from build123d import *

# Parameters (mm, degrees)
F1_DEPTH       = 10
F2_R           = 4.5
F3_R           = 1
F4_DEPTH       = 4
F5_R           = 2.4
F6_DEPTH       = 7.5
F3_R_2         = 2.4
F7_DEPTH       = 25
F7_DEPTH_BACK  = 25
F8_R           = 5
F9_R           = 1
F9_R_2         = 1.9
F10_DEPTH      = 25
F10_DEPTH_BACK = 25
F11_R          = 1


with BuildPart() as f1:
    # F0 (on Top) → F1 (new body)
    with BuildSketch(Plane.XY):
        Polygon((-22.5, 0), (0, 0), (22.5, 0), (22.5, 28.5), (19, 28.5), (19, 3.5), (0, 3.5), (-19, 3.5), (-19, 28.5), (-22.5, 28.5), align=None)
    extrude(amount=F1_DEPTH)

    # F2
    f2_edges = [f1.edges().sort_by_distance(p)[0] for p in [
        (-20.75, 28.5, 10),
        (-20.75, 28.5, 0),
        (20.75, 28.5, 10),
        (20.75, 28.5, 0),
    ]]
    fillet(f2_edges, radius=F2_R)

    # F3 (on face) → F4 (cut)
    with BuildSketch(Plane(origin=(-22.5, 0, 0), x_dir=(0, -1, 0), z_dir=(-1, 0, 0))):
        with Locations((-17, 5)):
            Circle(F3_R)
        with Locations((-11, 5)):
            Circle(F3_R)
    extrude(amount=-F4_DEPTH, mode=Mode.SUBTRACT)

    # F5 (on face) → F6 (join)
    with BuildSketch(Plane.YZ.offset(22.5)):
        with Locations((24, 5)):
            Circle(F5_R)
    extrude(amount=-F6_DEPTH)

    # F3 (on face) → F7 (cut, two sides)
    with BuildSketch(Plane(origin=(-22.5, 0, 0), x_dir=(0, -1, 0), z_dir=(-1, 0, 0))) as f7_sk:
        with Locations((-24, 5)):
            Circle(F3_R_2)
    extrude(amount=-F7_DEPTH, mode=Mode.SUBTRACT)
    extrude(f7_sk.sketch, amount=-F7_DEPTH_BACK, mode=Mode.SUBTRACT)

    # F8
    f8_edges = [f1.edges().sort_by_distance(p)[0] for p in [
        (-22.5, 0, 5),
        (22.5, 0, 5),
        (-19, 3.5, 5),
        (19, 3.5, 5),
    ]]
    fillet(f8_edges, radius=F8_R)

    # F9 (on face) → F10 (cut, two sides)
    with BuildSketch(Plane.XZ) as f10_sk:
        with Locations((-10.5, 5)):
            Circle(F9_R)
        with Locations((-2, 5)):
            Circle(F9_R_2)
        with Locations((6.5, 5)):
            Circle(F9_R)
    extrude(amount=-F10_DEPTH, mode=Mode.SUBTRACT)
    extrude(f10_sk.sketch, amount=-F10_DEPTH_BACK, mode=Mode.SUBTRACT)

    # F11
    f11_edges = [f1.edges().sort_by_distance(p)[0] for p in [
        (22.5, 14.5, 0),
        (21.035534, 1.464466, 0),
        (20.75, 24, 0),
        (0, 0, 0),
        (19, 16.25, 0),
        (-21.035534, 1.464466, 0),
        (17.535534, 4.964466, 0),
        (-22.5, 14.5, 0),
        (0, 3.5, 0),
        (-20.75, 24, 0),
        (-17.535534, 4.964466, 0),
        (-19, 16.25, 0),
    ]]
    fillet(f11_edges, radius=F11_R)


solid = f1.part
Verification items for the finished model (mm, model axes). A direction names the side the tool comes from. Round coordinates to 2 decimals unless told otherwise and drop trailing zeros. Loops run counter-clockwise (first coordinate to the right, second up) from the corner with the lowest first, then second, coordinate; pieces in that order, holes last. Notation, with made-up numbers: (60, 76.5) - (81, 76.5) arc R25 ccw to (81, 113.5) - close; hole circle Ø2 at (28.25, 26.5). An arc over 180 degrees is marked (long way). Use a Markdown table: item, result. Add a question column.
1. Release check for a two-part mould opening along X. For faces 1 (the face through (-22.215, 28.199, 4.993)), 2 (the face through (0, 0, 4)), 3 (the face through (-19.301, 16.358, 0.285)) record: released by +X, released by -X, zero draft, split by the parting line, or undercut.
2. Section check C-C, the plane x = 10. Record the boundary of the cut face in (y, z).
3. Access from +Z, -Z, +X, -X, +Y, -Y to the whole of each face (thin tool, end or side, straight path). Record for faces 4 (the face through (-0.196, 3.199, 0.285)), 5 (the face through (15, 24, 5)), 6 (the face through (19.301, 16.358, 9.715)).
4. Thickness scan on probe 1 along Z at (x, y) = (-2, 1.7); probe 2 along X at (y, z) = (19.5, 2.25); probe 3 along Z at (x, y) = (6.5, 1.9). Record the ranges inside material, lowest first. Write a range as [from, to].
5. Gauge pin test, flat ends, axial feed: pin 1 (4 mm diameter, centred on x = -6.5, z = 5.5, fed in from +Y); pin 2 (1.4 mm diameter, centred on y = 23.5, z = 4.5, fed in from -X); pin 3 (1.5 mm diameter, centred on x = 3.5, y = 4.5, fed in from -Z). Record the tip position at first contact, or that the pin passes through.
6. Section check B-B, the plane x = -2. Record the boundary of the cut face in (y, z), plus the area to 3 significant figures.
7. Section check A-A, the plane y = 19.25. Record the boundary of the cut face in (x, z), plus the area to 3 significant figures.
Checks:
| question | item | result |
|---|---|---|
| 1 | face 1 | released by -X |
| 1 | face 2 | zero draft |
| 1 | face 3 | undercut |
| 2 | outline | (0, 1) arc R1 ccw to (1, 0) - (2.5, 0) arc R1 ccw to (3.5, 1) - (3.5, 9) arc R1 ccw to (2.5, 10) - (1, 10) arc R1 ccw to (0, 9) - close |
| 3 | face 4 | -Z, +Y |
| 3 | face 5 | +Z, -Z, -X, +Y |
| 3 | face 6 | +Z, +Y |
| 4 | probe 1 | z = [0, 3.1], [6.9, 10] |
| 4 | probe 2 | x = [-22.5, -19], [19, 22.5] |
| 4 | probe 3 | z = [0, 4], [6, 10] |
| 5 | pin 1 | stops at y = 3.5 |
| 5 | pin 2 | stops at x = 15 |
| 5 | pin 3 | passes through |
| 6 | outline | (0, 1) arc R1 ccw to (1, 0) - (2.5, 0) arc R1 ccw to (3.5, 1) - (3.5, 3.1) - (0, 3.1) - close; (0, 6.9) - (3.5, 6.9) - (3.5, 9) arc R1 ccw to (2.5, 10) - (1, 10) arc R1 ccw to (0, 9) - close |
| 6 | area | 20.8 mm^2 |
| 7 | outline | (-22.5, 1) arc R1 ccw to (-21.5, 0) - (-20, 0) arc R1 ccw to (-19, 1) - (-19, 9) arc R1 ccw to (-20, 10) - (-21.5, 10) arc R1 ccw to (-22.5, 9) - close; (19, 1) arc R1 ccw to (20, 0) - (21.5, 0) arc R1 ccw to (22.5, 1) - (22.5, 9) arc R1 ccw to (21.5, 10) - (20, 10) arc R1 ccw to (19, 9) - close |
| 7 | area | 68.3 mm^2 |
